from build123d import *

# Parameters (mm, degrees)
BOSS_EXTRUDE1_DEPTH = 304.8
CUT_EXTRUDE1_DEPTH  = 12.7
SKETCH3_R           = 6.35
CUT_EXTRUDE2_DEPTH  = 12.7


with BuildPart() as part:
    # Sketch1 → Boss-Extrude1 (new body)
    with BuildSketch(Plane(origin=(0, 0, 0), x_dir=(1, 0, 0), z_dir=(0, 1, 0))):
        Polygon((-76.143480967, 44.082766217), (-63.443480967, 44.082766217), (-63.443480967, 70.416025302), (-30.342534375, 70.416025302), (-30.342534375, 83.116025302), (-76.143480967, 83.116025302), align=None)
    extrude(amount=BOSS_EXTRUDE1_DEPTH)

    # Sketch2 → Cut-Extrude1 (cut)
    with BuildSketch(Plane(origin=(0, 0, -83.116025302), x_dir=(-1, 0, 0), z_dir=(0, 0, -1))):
        with BuildLine():
            ThreePointArc((48.142771023, 11.450236648), (41.792771023, 17.800236648), (35.442771023, 11.450236648))
            Line((35.442771023, 11.450236648), (48.142771023, 11.450236648))
        make_face()
        with BuildLine():
            Line((48.142771023, 11.450236648), (35.442771023, 11.450236648))
            ThreePointArc((35.442771023, 11.450236648), (41.792771023, 5.100236648), (48.142771023, 11.450236648))
        make_face()
    extrude(amount=-CUT_EXTRUDE1_DEPTH, mode=Mode.SUBTRACT)

    # Sketch3 → Cut-Extrude2 (cut)
    with BuildSketch(Plane.ZY.offset(76.143480967)):
        with Locations((-53.841080989, 9.758314771)):
            Circle(SKETCH3_R)
    extrude(amount=-CUT_EXTRUDE2_DEPTH, mode=Mode.SUBTRACT)


solid = part.part
Can you work these out from the model? Positions are in its coordinate system, mm. A direction names the side the tool comes from. Give positions to 0.01 mm unless a question says otherwise; leave off trailing zeros. Loops run counter-clockwise (first coordinate to the right, second up) from the corner with the lowest first, then second, coordinate; pieces in that order, holes last. Notation, with made-up numbers: (-39.5, 8) - (2.5, 8) arc R20 ccw to (2.5, 47) - close; hole circle Ø11 at (-29.75, 61.25). An arc over 180 degrees is marked (long way). Answer as a JSON object with one key per item and string values.
Q1. Imagine slicing it at C-C on y = 270. Write out the boundary of the cut face in (x, z).
Geometry says:
{"outline": "(-76.14, -83.12) - (-30.34, -83.12) - (-30.34, -70.42) - (-63.44, -70.42) - (-63.44, -44.08) - (-76.14, -44.08) - close"}
Q2. Imagine slicing it at B-B on x = -41.5. Write out the boundary of the cut face in (y, z).
Geometry says:
{"outline": "(0, -83.12) - (5.11, -83.12) - (5.11, -70.42) - (0, -70.42) - close; (17.79, -83.12) - (304.8, -83.12) - (304.8, -70.42) - (17.79, -70.42) - close"}
Q3. If we mould it in two halves opening along Y, with no side actions, what happens to faces 3 (the cylindrical face through (-48.137, 11.171, -76.855)), 4 (the flat face through (-59, 0, -73)), 5 (the cylindrical face through (-69.88, 3.56, -55.22)), 6 (the flat face through (-70, 150, -44.083))? For each: pulls with the +Y half, pulls with the -Y half, needs draft (parallel to the pull), parting line crosses it, or undercut.
Geometry says:
{"face 3": "undercut", "face 4": "pulls with the -Y half", "face 5": "undercut", "face 6": "needs draft"}
Q4. Which directions (+Z, -Z, +X, -X, +Y, -Y) give clear straight access to the entire face, cutting with the end or side of a thin tool? Please do faces 1 (the flat face through (-47, 150, -70.416)), 2 (the flat face through (-59, 304.8, -73)).
Geometry says:
{"face 1": "+Z, +X, +Y, -Y", "face 2": "+Z, -Z, +X, -X, +Y"}
Q5. Imagine slicing it at D-D on z = -64. Write out the boundary of the cut face in (x, y).
Geometry says:
{"outline": "(-76.14, 0) - (-63.44, 0) - (-63.44, 304.8) - (-76.14, 304.8) - close"}
Q6. Will these pins go through, and if not, where does the flat tip stop? P1, Ø16.5, axis at x = -41.79, y = 11.45, coming from the +Z side; P2, Ø5, axis at x = -62, y = 221, coming from the +Z side; P3, Ø13, axis at y = 102.5, z = -56.5, coming from the +X side.
Geometry says:
{"P1": "z = -70.42", "P2": "z = -44.08", "P3": "x = -63.44"}
Q7. If I drill on L1, parallel to X at y = 285, z = -53; L2, parallel to Y at x = -67, z = -54; L3, parallel to Z at x = -37, y = 220.5, over which ranges is the centre line in solid material (lowest first)?
Geometry says:
{"L1": "-76.14 to -63.44", "L2": "0 to 3.41, 16.11 to 304.8", "L3": "-83.12 to -70.42"}
Q8. Imagine slicing it at A-A on z = -52. Write out the boundary of the cut face in (x, y), plus the area to 3 significant figures.
Geometry says:
{"outline": "(-76.14, 0) - (-63.44, 0) - (-63.44, 3.68) - (-76.14, 3.68) - close; (-76.14, 15.84) - (-63.44, 15.84) - (-63.44, 304.8) - (-76.14, 304.8) - close", "area": "3,720 mm²"}
